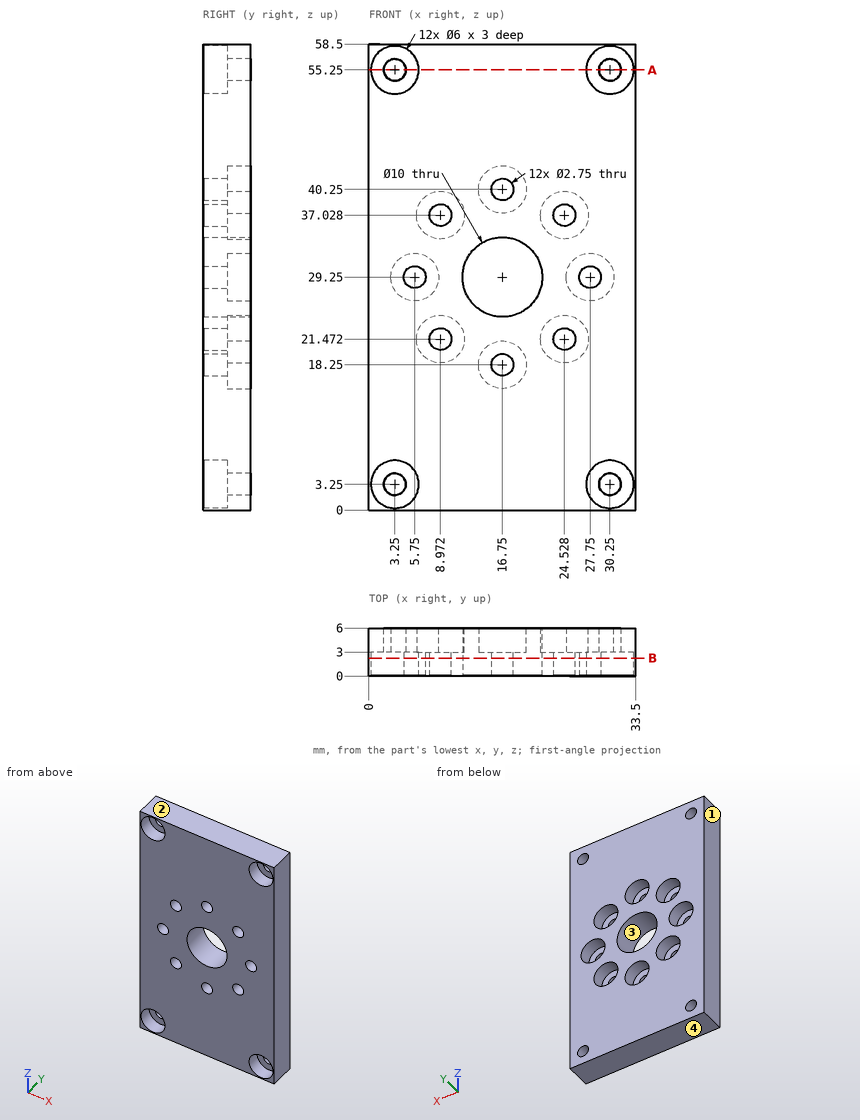
Answer from the drawing. Dimensions are ordinates in mm from the lowest x, y and z of the part. Give positions to 0.01 mm unless a question says otherwise; leave off trailing zeros. Loops run counter-clockwise (first coordinate to the right, second up) from the corner with the lowest first, then second, coordinate; pieces in that order, holes last.
Item 1: The part is cut by section A-A (z = 55.25). Write down the section's boundary in (x, y) (3 decimals), and give its area (4 significant figures).
Item 2: Each of these flat-tipped pins is pushed along its axis until it touches: pin 1 Ø3.5 at (x, z) = (27.75, 29.25) entering from +Y; pin 2 Ø1.8 at (x, z) = (31, 2.5) entering from -Y. Where does it stop, or does it pass through?
Item 3: Find the intervals of material crossed by line 1 along Z through (x, y) = (16.75, 4.85); line 2 along Z through (x, y) = (3.25, 0.75); line 3 along Z through (x, y) = (19, 5.5) (1 decimal), in increasing order.
Item 4: The mould has two halves that part along Z. Classify the marked faces 1, 2, 3 and 4: released by +Z, released by -Z, zero draft, split by the parting line, or undercut.
Item 5: The part is cut by section B-B (y = 2.25). Give the number of separate pieces and of enclosed holes in the cut face, and give its area (3 significant figures).
Taken from the geometry:
1. outline: (0, 0) - (0.25, 0) - (0.25, 3) - (1.875, 3) - (1.875, 6) - (0, 6) - close; (4.625, 3) - (6.25, 3) - (6.25, 0) - (27.25, 0) - (27.25, 3) - (28.875, 3) - (28.875, 6) - (4.625, 6) - close; (31.625, 3) - (33.25, 3) - (33.25, 0) - (33.5, 0) - (33.5, 6) - (31.625, 6) - close
1. area: 148.5 mm2
2. pin 1: stops at y = 3
2. pin 2: stops at y = 3
3. line 1: z = 0 to 15.25, 21.25 to 24.25, 34.25 to 37.25, 43.25 to 58.5
3. line 2: z = 0 to 0.25, 6.25 to 52.25, 58.25 to 58.5
3. line 3: z = 0 to 16.3, 20.2 to 24.8, 33.7 to 38.3, 42.2 to 58.5
4. face 1: zero draft
4. face 2: released by +Z
4. face 3: undercut
4. face 4: released by -Z
5. separate pieces: 1
5. enclosed holes: 13
5. area: 1,720 mm2
